Here's how the part is built. I have some questions about the finished solid (model axes, mm). Coordinates: 2 decimals unless noted, no trailing zeros. Loops run counter-clockwise (first coordinate to the right, second up) from the corner with the lowest first, then second, coordinate; pieces in that order, holes last. Notation, with made-up numbers: (81, 76.25) -> (108, 76.25) arc R17 cw to (108, 82.25) -> close; hole circle Ø3 at (59, 35.25). An arc over 180 degrees is marked (long way). Answer as a JSON object with one key per item and string values. Group by question number.
Q1. I want a section at B-B on z = 5.5. Write out the boundary of the cut face in (x, y) (3 decimals), then the cut area to 3 significant figures.
Q2. I want a section at D-D on x = 6. Write out the boundary of the cut face in (y, z), then the cut area to 3 significant figures.
Q3. I want a section at A-A on y = -5. Write out the boundary of the cut face in (x, z), then the cut area to 3 significant figures.
Q4. I want a section at C-C on x = 30.5. Write out the boundary of the cut face in (y, z).
Q5. I need wall thicknesses on line 1 (X direction, y = -25, z = 0.8); line 2 (Y direction, x = -42, z = 1.5); line 3 (Z direction, x = 28, y = 35). Which ranges of each line are inside material? Lowest first, please.
Q6. I'm going to push flat-ended pins straight in: pin 1 (1.5 mm diameter, centred on x = -33, y = 16.5, fed in from +Z); pin 2 (3 mm diameter, centred on x = -29.51, y = 35, fed in from -Z); pin 3 (4 mm diameter, centred on x = 30.49, y = 35, fed in from -Z). Where does each tip first touch, or does it pass through?
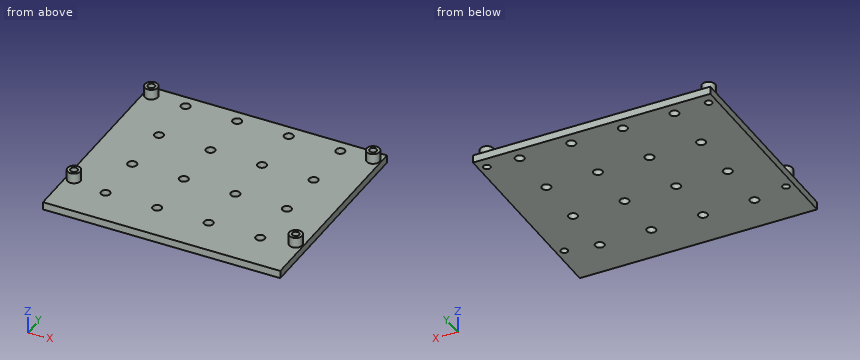
```python
from build123d import *

# Parameters (mm, degrees)
SKETCH1_W            = 92.024962686
SKETCH1_H            = 80
SKETCH1_R            = 1.365
BOSS_EXTRUDE1_DEPTH  = 3
SKETCH3_R            = 2.5
SKETCH3_R_2          = 1.365
BOSS_EXTRUDE2_DEPTH  = 4
CUT_EXTRUDE2_START   = -4
SKETCH4_R            = 1.75
CUT_EXTRUDE2_DEPTH   = 9
LPATTERN1_COUNT      = 4
LPATTERN1_PITCH      = 20
LPATTERN1_COUNT_DIR2 = 4
LPATTERN1_PITCH_DIR2 = 20


with BuildPart() as part:
    # Sketch1 → Boss-Extrude1 (new body)
    with BuildSketch(Plane.XY):
        Rectangle(SKETCH1_W, SKETCH1_H)
        with Locations((-42.997518657, 35.4)):
            Circle(SKETCH1_R, mode=Mode.SUBTRACT)
        with Locations((43.002481343, 35.4)):
            Circle(SKETCH1_R, mode=Mode.SUBTRACT)
        with Locations((-42.997518657, -22.6)):
            Circle(SKETCH1_R, mode=Mode.SUBTRACT)
        with Locations((43.002481343, -22.6)):
            Circle(SKETCH1_R, mode=Mode.SUBTRACT)
    extrude(amount=BOSS_EXTRUDE1_DEPTH)

    # Sketch3 → Boss-Extrude2 (add)
    with BuildSketch(Plane.XY.offset(3)):
        with Locations((-42.997518657, 35.4)):
            Circle(SKETCH3_R)
        with Locations((-42.997518657, 35.4)):
            Circle(SKETCH3_R_2, mode=Mode.SUBTRACT)
        with Locations((-42.997518657, -22.6)):
            Circle(SKETCH3_R)
        with Locations((-42.997518657, -22.6)):
            Circle(SKETCH3_R_2, mode=Mode.SUBTRACT)
        with Locations((43.002481343, 35.4)):
            Circle(SKETCH3_R)
        with Locations((43.002481343, 35.4)):
            Circle(SKETCH3_R_2, mode=Mode.SUBTRACT)
        with Locations((43.002481343, -22.6)):
            Circle(SKETCH3_R)
        with Locations((43.002481343, -22.6)):
            Circle(SKETCH3_R_2, mode=Mode.SUBTRACT)
    extrude(amount=BOSS_EXTRUDE2_DEPTH)

    # Sketch4 → Cut-Extrude2 (cut)
    with BuildSketch(Plane.XY.offset(3).offset(CUT_EXTRUDE2_START)):
        with Locations((-29.512481343, 35)):
            Circle(SKETCH4_R)
    cut_extrude2 = extrude(amount=CUT_EXTRUDE2_DEPTH, mode=Mode.SUBTRACT)

    # LPattern1: Cut-Extrude2 4 × 4
    with Locations(*[(i * LPATTERN1_PITCH, -j * LPATTERN1_PITCH_DIR2, 0) for i in range(LPATTERN1_COUNT) for j in range(LPATTERN1_COUNT_DIR2) if (i, j) != (0, 0)]):
        add(cut_extrude2, mode=Mode.SUBTRACT)


solid = part.part
```
Result set:
{
 "1": {"outline": "circle Ø5 at (-42.998, -22.6); circle Ø5 at (-42.998, 35.4); circle Ø5 at (43.002, -22.6); circle Ø5 at (43.002, 35.4); hole circle Ø2.73 at (-42.998, -22.6); hole circle Ø2.73 at (-42.998, 35.4); hole circle Ø2.73 at (43.002, -22.6); hole circle Ø2.73 at (43.002, 35.4)", "area": "55.1 mm²"},
 "2": {"outline": "(-40, 0) -> (40, 0) -> (40, 3) -> (-40, 3) -> close", "area": "240 mm²"},
 "3": {"outline": "(-46.01, 0) -> (-31.26, 0) -> (-31.26, 3) -> (-46.01, 3) -> close; (-27.76, 0) -> (-11.26, 0) -> (-11.26, 3) -> (-27.76, 3) -> close; (-7.76, 0) -> (8.74, 0) -> (8.74, 3) -> (-7.76, 3) -> close; (12.24, 0) -> (28.74, 0) -> (28.74, 3) -> (12.24, 3) -> close; (32.24, 0) -> (46.01, 0) -> (46.01, 3) -> (32.24, 3) -> close", "area": "234 mm²"},
 "4": {"outline": "(-40, 0) -> (-26.75, 0) -> (-26.75, 3) -> (-40, 3) -> close; (-23.25, 0) -> (-6.75, 0) -> (-6.75, 3) -> (-23.25, 3) -> close; (-3.25, 0) -> (13.25, 0) -> (13.25, 3) -> (-3.25, 3) -> close; (16.75, 0) -> (33.25, 0) -> (33.25, 3) -> (16.75, 3) -> close; (36.75, 0) -> (40, 0) -> (40, 3) -> (36.75, 3) -> close"},
 "5": {"line 1": "x = -46.01 to -31.26, -27.76 to -11.26, -7.76 to 8.74, 12.24 to 28.74, 32.24 to 46.01", "line 2": "y = -40 to -23.53, -21.67 to 34.47, 36.33 to 40", "line 3": "z = 0 to 3"},
 "6": {"pin 1": "stops at z = 3", "pin 2": "passes through", "pin 3": "stops at z = 0"}
}
